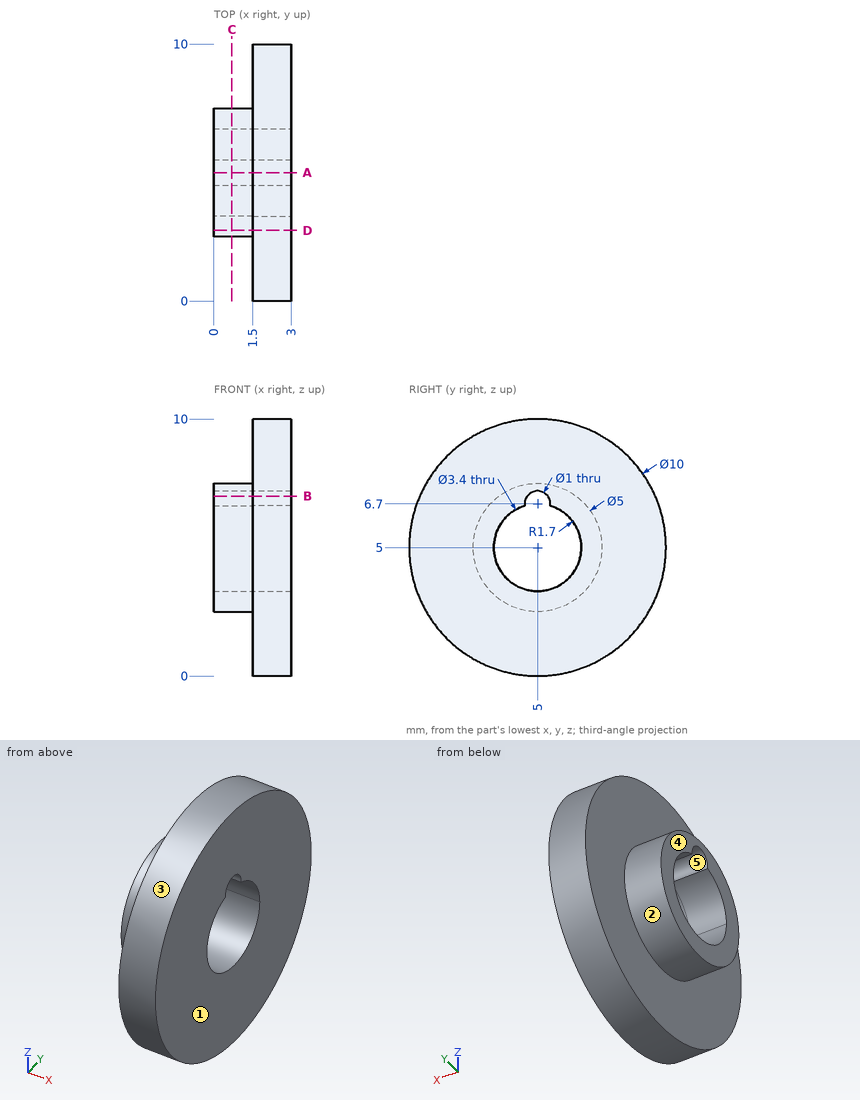
Check sheet for the drawn part. Datum: minimum x, y, z corner. Units: mm. A direction names the side the tool comes from. Round coordinates to 2 decimals unless told otherwise and drop trailing zeros. Order: outer loops, then holes, each group sorted by start corner. A loop starts at its lowest first (then second) coordinate and runs counter-clockwise, first axis right, second up. Notation, with made-up numbers: (28, -2.75) -> (36, -2.75) arc R33 ccw to (36, 32.25) -> close; hole circle Ø3 at (29.25, -26). An arc over 180 degrees is marked (long way). Use CSV: the item, a comma, the result in double quotes.
(1) Depth check by flat-ended pin: pin 1 (1 mm diameter, centred on x = 1.5, z = 7.5, fed in from +Y); pin 2 (3 mm diameter, centred on y = 5, z = 5, fed in from +X). Enter the tip coordinate at first touch or a pass-through.
Worked out:
pin 1,"y = 9.58"
pin 2,"through"
(2) Tool access check on the marked faces 1 and 2. Record the directions out of +Z, -Z, +X, -X, +Y, -Y that give a thin tool (end or side, any length) a straight path to the whole face; none if there is none.
Worked out:
face 1,"+Z, -Z, +X, +Y, -Y"
face 2,"-X"
(3) Draft check along Y on the marked faces 3, 4 and 5. Enter one of: pulls with the +Y half, pulls with the -Y half, needs draft (parallel to the pull), parting line crosses it, or undercut.
Worked out:
face 3,"parting line crosses it"
face 4,"needs draft"
face 5,"undercut"
(4) Cross-section at B-B (z = 7). Record the boundary of the cut face in (x, y).
Worked out:
outline,"(0, 3.5) -> (1.5, 3.5) -> (1.5, 0.42) -> (3, 0.42) -> (3, 4.6) -> (0, 4.6) -> close; (0, 5.4) -> (3, 5.4) -> (3, 9.58) -> (1.5, 9.58) -> (1.5, 6.5) -> (0, 6.5) -> close"
(5) Cross-section at C-C (x = 0.7). Record the boundary of the cut face in (y, z).
Worked out:
outline,"circle Ø5 at (5, 5); hole (4.51, 6.63) arc R1.7 ccw (long way) to (5.49, 6.63) arc R0.5 ccw (long way) to start"
(6) Cross-section at D-D (y = 2.75). Record the boundary of the cut face in (x, z).
Worked out:
outline,"(0, 3.91) -> (1.5, 3.91) -> (1.5, 0.53) -> (3, 0.53) -> (3, 9.47) -> (1.5, 9.47) -> (1.5, 6.09) -> (0, 6.09) -> close"
(7) Cross-section at A-A (y = 5). Record the boundary of the cut face in (x, z), and give its area (3 significant figures).
Worked out:
outline,"(0, 2.5) -> (1.5, 2.5) -> (1.5, 0) -> (3, 0) -> (3, 3.3) -> (0, 3.3) -> close; (0, 7.2) -> (3, 7.2) -> (3, 10) -> (1.5, 10) -> (1.5, 7.5) -> (0, 7.5) -> close"
area,"10.8 mm²"
(8) Material ranges on line 1 along Z through (x, y) = (2, 5); line 2 along X through (y, z) = (8.75, 7); line 3 along Z through (x, y) = (1.4, 5), recorded low to high. Write a range as from..to.
Worked out:
line 1,"0..3.3, 7.2..10"
line 2,"1.5..3"
line 3,"2.5..3.3, 7.2..7.5"
